Read the model definition and answer for the solid it produces. Units are mm, in the model's axes. A direction names the side the tool comes from. Give positions to 0.01 mm unless a question says otherwise; leave off trailing zeros. Order: outer loops, then holes, each group sorted by start corner. A loop starts at its lowest first (then second) coordinate and runs counter-clockwise, first axis right, second up. Notation, with made-up numbers: (-32.5, 43) - (-16.5, 43) arc R16 ccw to (-16.5, 54) - close; hole circle Ø8 at (42, 75). An arc over 180 degrees is marked (long way). Write item = value, one per line.
```python
from build123d import *

# Parameters (mm, degrees)
SKETCH1_R           = 25
BOSS_EXTRUDE1_DEPTH = 422.5
SKETCH2_R           = 10
CUT_EXTRUDE1_DEPTH  = 160
CUT_EXTRUDE3_DEPTH  = 5.5


with BuildPart() as part:
    # Sketch1 → Boss-Extrude1 (new, symmetric)
    with BuildSketch(Plane(origin=(0, 0, 0), x_dir=(0, 0, -1), z_dir=(1, 0, 0))):
        Circle(SKETCH1_R)
    extrude(amount=BOSS_EXTRUDE1_DEPTH, both=True)

    # Sketch2 → Cut-Extrude1 (cut, symmetric)
    with BuildSketch(Plane.XY):
        with Locations((392.5, 0)):
            Circle(SKETCH2_R)
        with Locations((272.5, 0)):
            Circle(SKETCH2_R)
    extrude(amount=CUT_EXTRUDE1_DEPTH, both=True, mode=Mode.SUBTRACT)

    # Sketch4 → Cut-Extrude3 (cut)
    with BuildSketch(Plane.XY.offset(25)):
        with BuildLine():
            Line((-422.5, 7), (-311.5, 7))
            ThreePointArc((-311.5, 7), (-304.5, 0), (-311.5, -7))
            Line((-311.5, -7), (-422.5, -7))
            ThreePointArc((-422.5, -7), (-429.5, 0), (-422.5, 7))
        make_face()
    extrude(amount=-CUT_EXTRUDE3_DEPTH, mode=Mode.SUBTRACT)


solid = part.part
```
1. Section D-D (x = -341.5) is taken. Determine the outline of the cut face in (y, z), and give its area (3 significant figures).
Recorded:
outline = (-7, 19.5) - (-7, 24) arc R25 ccw (long way) to (7, 24) - (7, 19.5) - close
area = 1,890 mm^2
2. Flat-ended cylindrical pins translate along their axes: pin 1 (2.5 mm diameter, centred on x = -379, z = 22.5, fed in from +Y); pin 2 (4 mm diameter, centred on x = 56, y = 11.5, fed in from +Z); pin 3 (6 mm diameter, centred on x = -235, y = -12, fed in from -Z). Find the tip coordinate at first contact, or state that the pin passes through.
Recorded:
pin_1 = 13.17
pin_2 = 23.12
pin_3 = -23.32
3. Section B-B (z = -17) is taken. Determine the outline of the cut face in (x, y), and give its area (3 significant figures).
Recorded:
outline = (-422.5, -18.33) - (422.5, -18.33) - (422.5, 18.33) - (-422.5, 18.33) - close; hole circle Ø20 at (272.5, 0); hole circle Ø20 at (392.5, 0)
area = 30,300 mm^2
4. Straight lines are drawn through the part: L1, parallel to X at y = 0, z = 2; L2, parallel to X at y = 2.5, z = -16; L3, parallel to Y at x = 329, z = -2.5. For each, find the intervals that lie inside material, in ascending order. Write a range as [from, to].
Recorded:
L1 = [-422.5, 262.5], [282.5, 382.5], [402.5, 422.5]
L2 = [-422.5, 262.82], [282.18, 382.82], [402.18, 422.5]
L3 = [-24.87, 24.87]
5. Determine the mould class of faces 1 (the face through (422.5, 0, 0)), 2 (the face through (5.915, 7.509, -23.846)), 3 (the face through (384.56, -6.08, 0.36)), 4 (the face through (282.04, 3, 0.36)) for opening direction Y: +Y half, -Y half, draft (parallel to the pull), parting line (faces both ways), or undercut.
Recorded:
face_1 = draft
face_2 = parting line
face_3 = undercut
face_4 = undercut
6. Section C-C (x = 272.5) is taken. Determine the outline of the cut face in (y, z), and give its area (3 significant figures).
Recorded:
outline = (-10, -22.91) - (-10, 22.91) arc R25 ccw to start; (10, -22.91) arc R25 ccw to (10, 22.91) - close
area = 991 mm^2
7. Section A-A (y = 0) is taken. Determine the outline of the cut face in (x, z).
Recorded:
outline = (-422.5, -25) - (262.5, -25) - (262.5, 25) - (-304.5, 25) - (-304.5, 19.5) - (-422.5, 19.5) - close; (282.5, -25) - (382.5, -25) - (382.5, 25) - (282.5, 25) - close; (402.5, -25) - (422.5, -25) - (422.5, 25) - (402.5, 25) - close
8. For faces 5 (the face through (-422.5, 0, 0)), 6 (the face through (-363, 0, 19.5)), determine the directions among +Z, -Z, +X, -X, +Y, -Y from which every point of the face is accessible in a straight line to the end or side of a thin tool.
Recorded:
face_5 = +Z, -Z, -X, +Y, -Y
face_6 = +Z, -X
